```python
from build123d import *


with BuildPart() as part:
    # Esquisse1 → Base-Révolution (revolve)
    with BuildSketch(Plane.XY, mode=Mode.PRIVATE) as base_r_volution_sk:
        with BuildLine():
            Line((-7, 104.5), (-3.598076211, 104.5))
            ThreePointArc((-3.598076211, 104.5), (-1, 106), (1.598076211, 104.5))
            Line((1.598076211, 104.5), (5, 104.5))
            Line((5, 104.5), (5, 107.5))
            ThreePointArc((5, 107.5), (4.707106781, 108.207106781), (4, 108.5))
            Line((4, 108.5), (-6, 108.5))
            ThreePointArc((-6, 108.5), (-6.707106781, 108.207106781), (-7, 107.5))
            Line((-7, 107.5), (-7, 104.5))
        make_face()
    revolve(base_r_volution_sk.sketch.rotate(Axis((-11.189264063, 87.5, 0), (1, 0, 0)), 90), axis=Axis((-11.189264063, 87.5, 0), (1, 0, 0)))


solid = part.part
```
Check sheet for the modelled part. Datum: model origin and axes. Units: mm. Give positions to 0.01 mm unless a question says otherwise; leave off trailing zeros. Write each loop counter-clockwise with the first axis right and the second up, starting at its lowest first coordinate (ties: lowest second). Pieces come first, ordered by that corner, then holes. Notation, with made-up numbers: (56, 77.5) - (71, 77.5) arc R11 cw to (71, 89.5) - close; hole circle Ø7 at (-1.5, 64.5). An arc over 180 degrees is marked (long way). Answer as a JSON object with one key per item and string values. Group by question number.
1) Sectioned sample at B-B (y = 87.5). Record the cut outline in (x, z).
2) Sectioned sample at A-A (z = 0). Record the cut outline in (x, y).
3) Release check for a two-part mould opening along Z. For faces 1 (the face through (-7, 102.2, -9)), 2 (the face through (-1.07, 106.13, 9.69)), 3 (the face through (-5.275, 104.096, -3.685)), 4 (the face through (3.323, 104.096, -3.685)) record: pulls with the +Z half, pulls with the -Z half, needs draft (parallel to the pull), parting line crosses it, or undercut.
4) Sectioned sample at C-C (x = 3). Record the cut outline in (y, z).
5) Thickness scan on probe 1 along Z at (x, y) = (3.15, 87.5); probe 2 along Y at (x, z) = (-3.75, 0); probe 3 along X at (y, z) = (79.5, -16). Record the ranges inside material, lowest first. Write a range as from..to.
6) Depth check by flat-ended pin: P1, Ø4, axis at x = -2.5, z = 15, coming from the +Y side; P2, Ø5, axis at x = -6, y = 81, coming from the -Z side; P3, Ø2, axis at x = 1, z = -10.5, coming from the -Y side; P4, Ø1.5, axis at y = 75, z = -9.5, coming from the +X side. Enter the tip coordinate at first touch or a pass-through.
Geometry results:
{
 "1": {"outline": "(-7, -20) arc R1 ccw to (-6, -21) - (4, -21) arc R1 ccw to (5, -20) - (5, -17) - (1.6, -17) arc R3 cw to (-3.6, -17) - (-7, -17) - close; (-7, 17) - (-3.6, 17) arc R3 cw to (1.6, 17) - (5, 17) - (5, 20) arc R1 ccw to (4, 21) - (-6, 21) arc R1 ccw to (-7, 20) - close"},
 "2": {"outline": "(-7, 67.5) arc R1 ccw to (-6, 66.5) - (4, 66.5) arc R1 ccw to (5, 67.5) - (5, 70.5) - (1.6, 70.5) arc R3 cw to (-3.6, 70.5) - (-7, 70.5) - close; (-7, 104.5) - (-3.6, 104.5) arc R3 cw to (1.6, 104.5) - (5, 104.5) - (5, 107.5) arc R1 ccw to (4, 108.5) - (-6, 108.5) arc R1 ccw to (-7, 107.5) - close"},
 "3": {"face 1": "needs draft", "face 2": "parting line crosses it", "face 3": "undercut", "face 4": "undercut"},
 "4": {"outline": "circle Ø42 at (87.5, 0); hole circle Ø34 at (87.5, 0)"},
 "5": {"probe 1": "z = -21..-17, 17..21", "probe 2": "y = 66.5..70.5, 104.5..108.5", "probe 3": "x = -7..-2.82, 0.82..5"},
 "6": {"P1": "stops at y = 103.99", "P2": "stops at z = -20.62", "P3": "stops at y = 68.77", "P4": "passes through"}
}
